Verification items for the finished model (mm, model axes). A direction names the side the tool comes from. Coordinates: 2 decimals unless noted, no trailing zeros. Order: outer loops, then holes, each group sorted by start corner. A loop starts at its lowest first (then second) coordinate and runs counter-clockwise, first axis right, second up.
Q1. Cross-section at A-A, the plane z = 0.5. Record the boundary of the cut face in (x, y).
Q2. Cross-section at B-B, the plane y = 14. Record the boundary of the cut face in (x, z), and give its area (3 significant figures).
Q3. Set-up check for faces 4 (the flat face through (6, 14, 2)), 5 (the flat face through (15, 12.95, 1)): record each of +Z, -Z, +X, -X, +Y, -Y from which the full face is reachable in a straight line by a thin tool's end or side.
Q4. Depth check by flat-ended pin: P1, Ø0.6, axis at x = 16, z = 1.5, coming from the +Y side; P2, Ø8, axis at x = 0, y = 14, coming from the +Z side; P3, Ø1, axis at x = -16.5, z = 1.5, coming from the +Y side. Enter the tip coordinate at first touch or a pass-through.
Q5. Thickness scan on line 1 (Y direction, x = 0, z = 1.3); line 2 (X direction, y = 10, z = 1.7); line 3 (Y direction, x = 16.5, z = 0.15). Record the ranges inside material, lowest first.
Q6. Draft check along Y on faces 1 (the flat face through (10.95, 14, 1)), 2 (the cylindrical face through (-6.395, -14.799, 0.986)), 3 (the flat face through (6, 14, 0)). Enter one of: pulls with the +Y half, pulls with the -Y half, needs draft (parallel to the pull), parting line crosses it, or undercut.
Q7. Cross-section at D-D, the plane x = -14. Record the boundary of the cut face in (y, z), and give its area (3 significant figures).
Q8. Cross-section at C-C, the plane x = 0. Record the boundary of the cut face in (y, z).
from build123d import *

# Parameters (mm, degrees)
SKETCH_1_R      = 29.5
SKETCH_1_R_2    = 2.05
SKETCH_1_R_3    = 5.05
SKETCH_1_W      = 8.1
SKETCH_1_H      = 2.1
EXTRUDE_1_DEPTH = 2


with BuildPart() as part:
    # 草图1 → 凸台-拉伸1 (new body)
    with BuildSketch(Plane.XY):
        with Locations((0, 14)):
            Circle(SKETCH_1_R)
        Circle(SKETCH_1_R_2, mode=Mode.SUBTRACT)
        with Locations((0, 14)):
            Circle(SKETCH_1_R_3, mode=Mode.SUBTRACT)
        with Locations((-15, 14)):
            Rectangle(SKETCH_1_W, SKETCH_1_H, mode=Mode.SUBTRACT)
        with Locations((15, 14)):
            Rectangle(SKETCH_1_W, SKETCH_1_H, mode=Mode.SUBTRACT)
    extrude(amount=EXTRUDE_1_DEPTH)


solid = part.part
Check values:
1. outline: circle Ø59 at (0, 14); hole (-19.05, 12.95) - (-10.95, 12.95) - (-10.95, 15.05) - (-19.05, 15.05) - close; hole circle Ø10.1 at (0, 14); hole circle Ø4.1 at (0, 0); hole (10.95, 12.95) - (19.05, 12.95) - (19.05, 15.05) - (10.95, 15.05) - close
2. outline: (-29.5, 0) - (-19.05, 0) - (-19.05, 2) - (-29.5, 2) - close; (-10.95, 0) - (-5.05, 0) - (-5.05, 2) - (-10.95, 2) - close; (5.05, 0) - (10.95, 0) - (10.95, 2) - (5.05, 2) - close; (19.05, 0) - (29.5, 0) - (29.5, 2) - (19.05, 2) - close
2. area: 65.4 mm2
3. face 4: +Z, +X, -X, +Y, -Y
3. face 5: +Z, -Z
4. P1: stops at y = 38.98
4. P2: passes through
4. P3: stops at y = 38.78
5. line 1: y = -15.5 to -2.05, 2.05 to 8.95, 19.05 to 43.5
5. line 2: x = -29.23 to -3.08, 3.08 to 29.23
5. line 3: y = -10.45 to 12.95, 15.05 to 38.45
6. face 1: undercut
6. face 2: parting line crosses it
6. face 3: needs draft
7. outline: (-11.97, 0) - (12.95, 0) - (12.95, 2) - (-11.97, 2) - close; (15.05, 0) - (39.97, 0) - (39.97, 2) - (15.05, 2) - close
7. area: 99.7 mm2
8. outline: (-15.5, 0) - (-2.05, 0) - (-2.05, 2) - (-15.5, 2) - close; (2.05, 0) - (8.95, 0) - (8.95, 2) - (2.05, 2) - close; (19.05, 0) - (43.5, 0) - (43.5, 2) - (19.05, 2) - close
